Here's how the part is built. I have some questions about the finished solid (model axes, mm). A direction names the side the tool comes from. Round coordinates to 2 decimals unless told otherwise and drop trailing zeros. Write each loop counter-clockwise with the first axis right and the second up, starting at its lowest first coordinate (ties: lowest second). Pieces come first, ordered by that corner, then holes. Notation, with made-up numbers: M 0,-11 L 59,-11 A14 cw 59,7 Z; hole C 31.5,-25 d3. An arc over 180 degrees is marked long. Write item = value, one per line. Start each with the question number.
(1) I want a section at A-A (z = -5). List the corners of the cut face in (x, y) for me.
(2) On a 3-axis mill with a long thin cutter (end or side, diameter ignored), from which of +Z, -Z, +X, -X, +Y, -Y can I reach the whole of each face in a straight line? I mean faces 1 (the flat face through (25.4, 7, -3.6)), 2 (the flat face through (7, 5, -19.9)), 3 (the cylindrical face through (39.28, 5.97, -14.43)), 4 (the flat face through (20, 5, 0)), 5 (the flat face through (20, 0, -13)). Say none if no direction works.
(3) Will these pins go through, and if not, where does the flat tip stop? pin 1 Ø3 at (x, z) = (24, -21.5) entering from +Y; pin 2 Ø1.6 at (y, z) = (5, -21.5) entering from -X; pin 3 Ø5 at (x, y) = (9.5, 7) entering from -Z.
(4) I want a section at B-B (x = 24). List the corners of the cut face in (y, z) for me.
(5) I want a section at C-C (y = 5). List the corners of the cut face in (x, z) for me.
(6) I want a section at D-D (z = -17.5). List the corners of the cut face in (x, y) for me, and give its area (3 significant figures).
(7) I need wall thicknesses on line 1 along Z through (x, y) = (24, 9.1); line 2 along X through (y, z) = (5, -13.75); line 3 along X through (y, z) = (5.25, -5). Which ranges of each line are inside material? Lowest first, please.
(8) If we mould it in two halves opening along X, with no side actions, what happens to faces 6 (the cylindrical face through (0.301, 5.07, -19.615)), 7 (the flat face through (28, 5, -25)), 8 (the flat face through (25.4, 7, -18.6)), 9 (the cylindrical face through (40.225, 5.07, -24.699))? For each: released by +X, released by -X, zero draft, split by the parting line, or undercut.
```python
from build123d import *

# Parameters (mm, degrees)
BOSS_EXTRUDE1_DEPTH            = 10
FILLET1_R                      = 1
CBORE_FOR_M3_SHCS1_D           = 3.4
CBORE_FOR_M3_SHCS1_DEPTH       = 10
CBORE_FOR_M3_SHCS1_CBORE_D     = 6.5
CBORE_FOR_M3_SHCS1_CBORE_DEPTH = 3
SKETCH5_R                      = 1.15
CUT_EXTRUDE1_DEPTH             = 2.5


with BuildPart() as part:
    # Sketch1 → Boss-Extrude1 (new body)
    with BuildSketch(Plane(origin=(0, 0, 0), x_dir=(1, 0, 0), z_dir=(0, 1, 0))):
        Polygon((0, 0), (40.51, 0), (40.51, 25), (14.6, 25), (14.6, 19.9), (0, 19.9), align=None)
    extrude(amount=BOSS_EXTRUDE1_DEPTH)

    # Fillet1
    fillet1_edges = [part.edges().sort_by_distance(p)[0] for p in [
        (0, 5, -19.9),
        (14.6, 5, -19.9),
        (14.6, 5, -25),
        (40.51, 5, -25),
        (40.51, 5, 0),
        (0, 5, 0),
    ]]
    fillet(fillet1_edges, radius=FILLET1_R)

    # CBORE for M3 SHCS1
    with Locations(Plane(origin=(0, 10, 0), x_dir=(1, 0, 0), z_dir=(0, 1, 0))):
        with Locations((24, 20), (24, 5)):
            CounterBoreHole(CBORE_FOR_M3_SHCS1_D / 2, CBORE_FOR_M3_SHCS1_CBORE_D / 2, CBORE_FOR_M3_SHCS1_CBORE_DEPTH, depth=CBORE_FOR_M3_SHCS1_DEPTH)

    # Sketch5 → Cut-Extrude1 (cut, symmetric)
    with BuildSketch(Plane(origin=(40.51, 0, 0), x_dir=(0, 0, -1), z_dir=(1, 0, 0))):
        with Locations((13.81, 5)):
            Circle(SKETCH5_R)
    extrude(amount=CUT_EXTRUDE1_DEPTH, both=True, mode=Mode.SUBTRACT)


solid = part.part
```
Returned:
q1.outline = M 0,0 L 22.3,0 L 22.3,7 L 20.75,7 L 20.75,10 L 0,10 Z; M 25.7,0 L 40.51,0 L 40.51,10 L 27.25,10 L 27.25,7 L 25.7,7 Z
q2.face_1 = +Y
q2.face_2 = -Z, -X, +Y, -Y
q2.face_3 = +X
q2.face_4 = +Z, +X, -X, +Y, -Y
q2.face_5 = +Z, -Z, +X, -X, -Y
q3.pin_1 = 7
q3.pin_2 = 14.58
q3.pin_3 = -19.9
q4.outline = M 0,-25 L 10,-25 L 10,-23.25 L 7,-23.25 L 7,-21.7 L 0,-21.7 Z; M 0,-18.3 L 7,-18.3 L 7,-16.75 L 10,-16.75 L 10,-8.25 L 7,-8.25 L 7,-6.7 L 0,-6.7 Z; M 0,-3.3 L 7,-3.3 L 7,-1.75 L 10,-1.75 L 10,0 L 0,0 Z
q5.outline = M 0,-18.9 A1 ccw 1,-19.9 L 13.6,-19.9 A1 cw 14.6,-20.9 L 14.6,-24 A1 ccw 15.6,-25 L 39.51,-25 A1 ccw 40.51,-24 L 40.51,-14.96 L 38.01,-14.96 L 38.01,-12.66 L 40.51,-12.66 L 40.51,-1 A1 ccw 39.51,0 L 1,0 A1 ccw 0,-1 Z; hole C 24,-20 d3.4; hole C 24,-5 d3.4
q6.outline = M 0,0 L 40.51,0 L 40.51,10 L 26.08,10 L 26.08,7 L 21.92,7 L 21.92,10 L 0,10 Z
q6.area = 393 mm²
q7.line_1 = -25 to -23.25, -16.75 to -8.25, -1.75 to 0
q7.line_2 = 0 to 38.01
q7.line_3 = 0 to 22.3, 25.7 to 40.51
q8.face_6 = released by -X
q8.face_7 = zero draft
q8.face_8 = undercut
q8.face_9 = released by +X
